```python
from build123d import *

# Parameters (mm, degrees)
F0_R     = 12.37214
F1_DEPTH = 10


with BuildPart() as f1:
    # F0 (on Top) → F1 (new body)
    with BuildSketch(Plane.XY):
        with BuildLine():
            Line((0, 40.147543), (0, 0))
            Line((0, 0), (55.64775, 0))
            Line((55.64775, 0), (55.64775, 30.147543))
            ThreePointArc((55.64775, 30.147543), (52.718818, 37.218611), (45.64775, 40.147543))
            Line((45.64775, 40.147543), (0, 40.147543))
        make_face()
        with Locations((26.765032, 18.186493)):
            Circle(F0_R, mode=Mode.SUBTRACT)
    extrude(amount=F1_DEPTH)


solid = f1.part
```
CAD build for the part. Positions are in the model's coordinates, mm. Give positions to 0.01 mm unless a question says otherwise; leave off trailing zeros. Write each loop counter-clockwise with the first axis right and the second up, starting at its lowest first coordinate (ties: lowest second). Pieces come first, ordered by that corner, then holes. Notation, with made-up numbers: M 19.25,-25.5 L 47.25,-25.5 A25 cw 47.25,4.5 Z; hole C 0,-30.5 d8. An arc over 180 degrees is marked long. Return JSON: item names as keys, results as strings. Group by question number.
(1) Band-saw the part on B-B (y = 13.5). Give the cut face in (x, z), and give its area (3 significant figures).
(2) Band-saw the part on C-C (z = 2.25). Give the cut face in (x, y).
(3) Drill centre lines: L1, parallel to Y at x = 26.5, z = 5.25; L2, parallel to Y at x = 28, z = 5.75; L3, parallel to X at y = 12.5, z = 8.5. Where is each one in solid material? Low to high. Write a range as [from, to].
(4) Band-saw the part on A-A (x = 33.5). Give the cut face in (y, z).
(5) Mould opens along X. For faces 1 (the face through (23, 40.148, 5)), 2 (the face through (55.648, 15, 5)), 3 (the face through (0, 20, 5)), 4 (the face through (25.154, 30.453, 4.93)) say: pulls with the +X half, pulls with the -X half, needs draft (parallel to the pull), parting line crosses it, or undercut.
Entries:
{
 "1": {"outline": "M 0,0 L 15.31,0 L 15.31,10 L 0,10 Z; M 38.22,0 L 55.65,0 L 55.65,10 L 38.22,10 Z", "area": "327 mm^2"},
 "2": {"outline": "M 0,0 L 55.65,0 L 55.65,30.15 A10 ccw 45.65,40.15 L 0,40.15 Z; hole C 26.77,18.19 d24.74"},
 "3": {"L1": "y = [0, 5.82], [30.56, 40.15]", "L2": "y = [0, 5.88], [30.5, 40.15]", "L3": "x = [0, 15.78], [37.75, 55.65]"},
 "4": {"outline": "M 0,0 L 7.81,0 L 7.81,10 L 0,10 Z; M 28.56,0 L 40.15,0 L 40.15,10 L 28.56,10 Z"},
 "5": {"face 1": "needs draft", "face 2": "pulls with the +X half", "face 3": "pulls with the -X half", "face 4": "undercut"}
}
